Could you check a few things on this model? Use its own coordinates, in mm. A direction names the side the tool comes from. Coordinates: 2 decimals unless noted, no trailing zeros. Write each loop counter-clockwise with the first axis right and the second up, starting at its lowest first coordinate (ties: lowest second). Pieces come first, ordered by that corner, then holes.
Item 1: I want a section at C-C on z = 5. Please give me the cut outline in (x, y).
Item 2: I want a section at B-B on x = 0. Please give me the cut outline in (y, z), then the cut area to 3 significant figures.
Item 3: I want a section at D-D on z = -4.5. Please give me the cut outline in (x, y).
Item 4: Thinking about a two-plate mould opening in X: for faces 3 (the cylindrical face through (3.233, 2.958, 1.341)), 4 (the flat face through (4, 0, 0)), 5 (the cylindrical face through (4.57, 5.24, -7.167)), which applies, +X half, -X half, draft (parallel to the pull), parting line (faces both ways), or undercut?
Item 5: I want a section at A-A on z = 0. Please give me the cut outline in (x, y), then the cut area to 3 significant figures.
Item 6: If I drill on probe 1 along X at (y, z) = (2.9, 0); probe 2 along Y at (x, z) = (-6.5, 3.25), over which ranges is the centre line in solid material (lowest first)?
Item 7: Which directions (+Z, -Z, +X, -X, +Y, -Y) give clear straight access to the entire face, cutting with the end or side of a thin tool? Please do faces 1 (the flat face through (4, 6, 0)), 2 (the flat face through (6, 1.5, 4)).
Item 8: For P1, Ø8, axis at x = 2.5, z = -4, coming from the -Y side; P2, Ø1.5, axis at y = 1, z = -4.5, coming from the +X side, each with a flat end and sliding along its axis, tell me the tip position at first contact or that it passes through.
from build123d import *

# Parameters (mm, degrees)
SKIZZE1_R                       = 8.5
SKIZZE1_R_2                     = 3.5
AUFSATZ_LINEAR_AUSTRAGEN1_DEPTH = 6
SCHNITT_LINEAR_START            = 1.5
SKIZZE2_R                       = 13.890066822
SKIZZE2_R_2                     = 6.709730291
SCHNITT_LINEAR_AUSTRAGEN1_DEPTH = 3


with BuildPart() as part:
    # Skizze1 → Aufsatz-Linear austragen1 (new body)
    with BuildSketch(Plane(origin=(0, 0, 0), x_dir=(1, 0, 0), z_dir=(0, 1, 0))):
        Circle(SKIZZE1_R)
        Circle(SKIZZE1_R_2, mode=Mode.SUBTRACT)
    extrude(amount=AUFSATZ_LINEAR_AUSTRAGEN1_DEPTH)

    # Skizze2 → Schnitt-Linear austragen1 (cut)
    with BuildSketch(Plane(origin=(0, 0, 0), x_dir=(1, 0, 0), z_dir=(0, 1, 0)).offset(SCHNITT_LINEAR_START)):
        Circle(SKIZZE2_R)
        Circle(SKIZZE2_R_2, mode=Mode.SUBTRACT)
    extrude(amount=SCHNITT_LINEAR_AUSTRAGEN1_DEPTH, mode=Mode.SUBTRACT)


solid = part.part
Response values:
1. outline: (-6.87, 0) - (6.87, 0) - (6.87, 1.5) - (4.47, 1.5) - (4.47, 4.5) - (6.87, 4.5) - (6.87, 6) - (-6.87, 6) - (-6.87, 4.5) - (-4.47, 4.5) - (-4.47, 1.5) - (-6.87, 1.5) - close
2. outline: (0, -8.5) - (1.5, -8.5) - (1.5, -6.71) - (4.5, -6.71) - (4.5, -8.5) - (6, -8.5) - (6, -3.5) - (0, -3.5) - close; (0, 3.5) - (6, 3.5) - (6, 8.5) - (4.5, 8.5) - (4.5, 6.71) - (1.5, 6.71) - (1.5, 8.5) - (0, 8.5) - close
2. area: 49.3 mm2
3. outline: (-7.21, 0) - (7.21, 0) - (7.21, 1.5) - (4.98, 1.5) - (4.98, 4.5) - (7.21, 4.5) - (7.21, 6) - (-7.21, 6) - (-7.21, 4.5) - (-4.98, 4.5) - (-4.98, 1.5) - (-7.21, 1.5) - close
4. face 3: undercut
4. face 4: draft
4. face 5: parting line
5. outline: (-8.5, 0) - (-3.5, 0) - (-3.5, 6) - (-8.5, 6) - (-8.5, 4.5) - (-6.71, 4.5) - (-6.71, 1.5) - (-8.5, 1.5) - close; (3.5, 0) - (8.5, 0) - (8.5, 1.5) - (6.71, 1.5) - (6.71, 4.5) - (8.5, 4.5) - (8.5, 6) - (3.5, 6) - close
5. area: 49.3 mm2
6. probe 1: x = -6.71 to -3.5, 3.5 to 6.71
6. probe 2: y = 0 to 1.5, 4.5 to 6
7. face 1: +Z, -Z, +X, -X, +Y
7. face 2: none
8. P1: stops at y = 0
8. P2: stops at x = 7.63
